Answer from the drawing. Dimensions are ordinates in mm from the lowest x, y and z of the part. A direction names the side the tool comes from. Give positions to 0.01 mm unless a question says otherwise; leave off trailing zeros. Loops run counter-clockwise (first coordinate to the right, second up) from the corner with the lowest first, then second, coordinate; pieces in that order, holes last. Notation, with made-up numbers: M -35.75,-39.5 L 3.25,-39.5 A33 cw 3.25,-8.5 Z; hole C 56,46 d4. An arc over 180 degrees is marked long. Use a Markdown table: item, result.
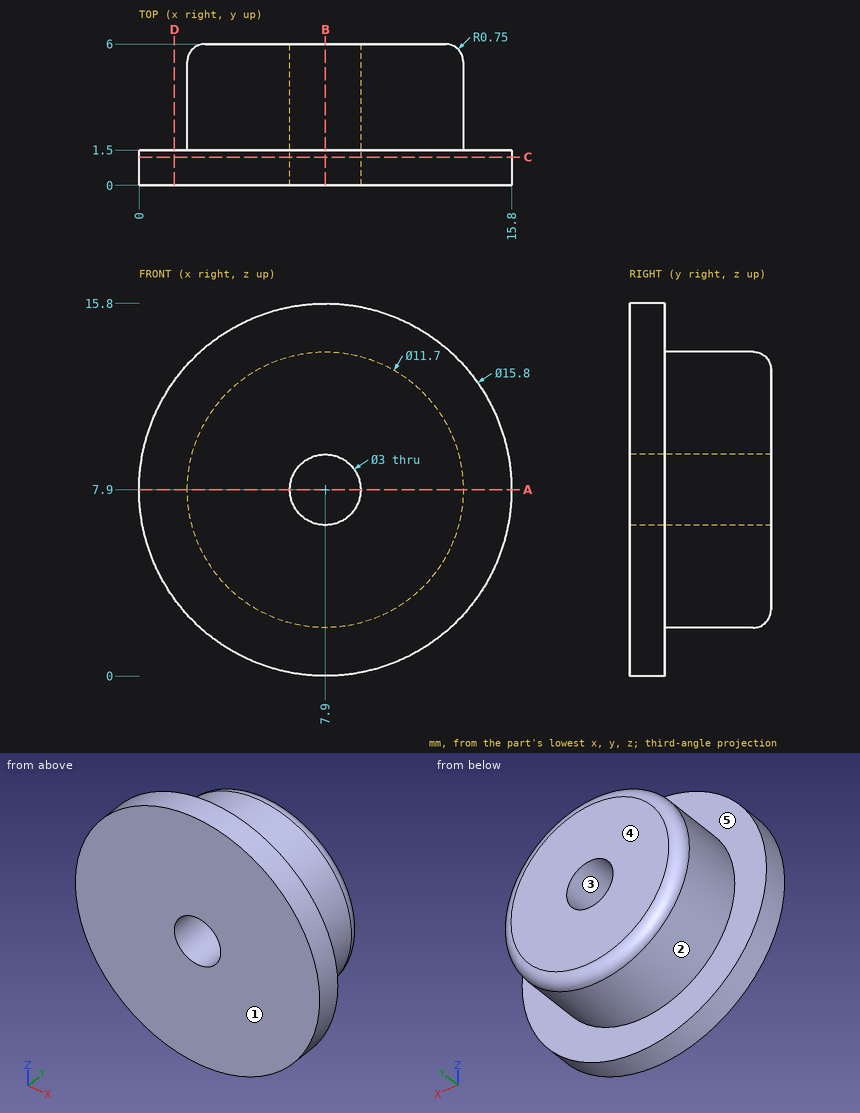
(1) Consider probe 1 along Z at (x, y) = (7.9, 2.4); probe 2 along Z at (x, y) = (7.9, 1.3); probe 3 along Y at (x, z) = (4.75, 2.5). Determine where each line is inside the solid, lowest interval first. Write a range as [from, to].
Entries:
| item | result |
|---|---|
| probe 1 | z = [2.05, 6.4], [9.4, 13.75] |
| probe 2 | z = [0, 6.4], [9.4, 15.8] |
| probe 3 | y = [0, 1.5] |
(2) Given P1, Ø6, axis at x = 13.5, z = 14, coming from the +Y side; P2, Ø1, axis at x = 4, y = 3.5, coming from the -Z side, each flat-ended and moving along its own axis, determine where each tip first touches the part or whether it passes through.
Entries:
| item | result |
|---|---|
| P1 | stops at y = 5.98 |
| P2 | stops at z = 3.14 |
(3) A cutting plane is placed at B-B (x = 7.9). Write down the section's boundary in (y, z).
Entries:
| item | result |
|---|---|
| outline | M 0,0 L 1.5,0 L 1.5,2.05 L 5.25,2.05 A0.75 ccw 6,2.8 L 6,6.4 L 0,6.4 Z; M 0,9.4 L 6,9.4 L 6,13 A0.75 ccw 5.25,13.75 L 1.5,13.75 L 1.5,15.8 L 0,15.8 Z |
(4) Which of the six approach directions +Z, -Z, +X, -X, +Y, -Y give full straight-line access (tool end or side, diameter ignored) to the marked faces 4 and 5?
Entries:
| item | result |
|---|---|
| face 4 | +Z, -Z, +X, -X, +Y |
| face 5 | +Y |
(5) A cutting plane is placed at C-C (y = 1.2). Write down the section's boundary in (x, z).
Entries:
| item | result |
|---|---|
| outline | C 7.9,7.9 d15.8; hole C 7.9,7.9 d3 |
(6) The mould has two halves that part along Z. Classify the marked faces 1, 2 and 3: released by +Z, released by -Z, zero draft, split by the parting line, or undercut.
Entries:
| item | result |
|---|---|
| face 1 | zero draft |
| face 2 | split by the parting line |
| face 3 | undercut |
(7) A cutting plane is placed at A-A (z = 7.9). Write down the section's boundary in (x, y), and give its area (3 significant figures).
Entries:
| item | result |
|---|---|
| outline | M 0,0 L 6.4,0 L 6.4,6 L 2.8,6 A0.75 ccw 2.05,5.25 L 2.05,1.5 L 0,1.5 Z; M 9.4,0 L 15.8,0 L 15.8,1.5 L 13.75,1.5 L 13.75,5.25 A0.75 ccw 13,6 L 9.4,6 Z |
| area | 58.1 mm² |
(8) A cutting plane is placed at D-D (x = 1.5). Write down the section's boundary in (y, z), and give its area (3 significant figures).
Entries:
| item | result |
|---|---|
| outline | M 0,3.27 L 1.5,3.27 L 1.5,12.53 L 0,12.53 Z |
| area | 13.9 mm² |
